Could you check a few things on this model? Use its own coordinates, in mm. Face numbers are marked on the shaded views. A direction names the side the tool comes from. Coordinates: 2 decimals unless noted, no trailing zeros. Order: outer loops, then holes, each group sorted by start corner. A loop starts at its lowest first (then second) coordinate and runs counter-clockwise, first axis right, second up. Notation, with made-up numbers: (-21, 45) - (17, 45) arc R24 cw to (17, 78) - close; hole circle Ø10 at (85, 10.25). An arc over 180 degrees is marked (long way). One line per item, written item: value.
Autodesk Inventor part; units mm, degrees
ref_plane "YZ Plane" through (0, 0, 0) normal (1, 0, 0) x (0, 1, 0)
ref_plane "XZ Plane" through (0, 0, 0) normal (0, 1, 0) x (-1, 0, 0)
ref_plane "XY Plane" through (0, 0, 0) normal (0, 0, 1) x (1, 0, 0)
sketch "Эскиз1" plane through (0, 0, 0) normal (0, 0, 1) x (1, 0, 0)
  circle A0 centre (0, 0) radius 2.1
  line L0 (-5, 14.35) -> (5, 14.35)
  line L1 (5, 14.35) -> (5, -14.35)
  line L2 (5, -14.35) -> (-5, -14.35)
  line L3 (-5, -14.35) -> (-5, 14.35)
  line L4 (-5, 14.35) -> (5, -14.35) construction
  line L5 (5, 14.35) -> (-5, -14.35) construction
  line L6 (-5, 7) -> (5, 7)
  dimension "d0" = 4.2
  dimension "d2" = 10
  dimension "d3" = 28.7
  dimension "d4" = 7
extrude "Выдавливание1" add sketch "Эскиз1" along normal blind 3.2 contours L6 L1 L2 L3
sketch "Эскиз2" plane through (0, 0, 3.2) normal (0, 0, 1) x (1, 0, 0)
  line L0 (5, -14.35) -> (5, 7)
  line L1 (5, -14.35) -> (-5, -14.35)
  line L2 (-5, -14.35) -> (-5, -11.15)
  line L3 (-5, -11.15) -> (5, -11.15)
  line L4 (5, -11.15) -> (5, -14.35)
  point P0 (0, 0)
  point P1 (5, -11.15)
  dimension "d7" = 10
  dimension "d8" = 3.2
extrude "Выдавливание2" add sketch "Эскиз2" along normal blind 13
fillet "Сопряжение1" radius 3 1 edges at (0, -11.15, 3.2)
sketch "Эскиз3" plane through (-5, -11.15, 16.2) normal (0, 1, 0) x (1, 0, 0)
  line L0 (0, 10) -> (10, 10)
  line L1 (5, 10) -> (5, 0)
  line L2 (0, 0) -> (10, 0)
  circle A0 centre (5, 5) radius 2.1
  point P0 (5, 16.2)
  dimension "d12" = 4.2
extrude "Выдавливание3" cut sketch "Эскиз3" against normal blind 13
sketch "Эскиз4" plane through (5, -14.35, 0) normal (1, 0, 0) x (0, 0, -1)
  line L0 (0, 0) -> (0, 21.35)
  line L1 (0, 21.35) -> (-3.2, 21.35)
  line L2 (-3.2, 6.2) -> (-3.2, 21.35)
  arc A0 (-6.2, 3.2) -> (-3.2, 6.2) centre (-6.2, 6.2) ccw
  line L3 (-6.2, 3.2) -> (-16.2, 3.2)
  line L4 (-16.2, 0) -> (-16.2, 3.2)
  line L5 (0, 0) -> (-16.2, 0)
  point P0 (0, 14.35)
extrude "Выдавливание4" add sketch "Эскиз4" along normal blind 3
sketch "Эскиз5" plane through (-5, -14.35, 0) normal (-1, 0, 0) x (0, 0, 1)
  line L0 (0, 21.35) -> (0, 0)
  line L1 (0, 0) -> (16.2, 0)
  line L2 (16.2, 3.2) -> (16.2, 0)
  line L3 (6.2, 3.2) -> (16.2, 3.2)
  arc A0 (3.2, 6.2) -> (6.2, 3.2) centre (6.2, 6.2) ccw
  line L4 (3.2, 21.35) -> (3.2, 6.2)
  line L5 (0, 21.35) -> (3.2, 21.35)
  point P0 (0, 14.35)
extrude "Выдавливание5" add sketch "Эскиз5" along normal blind 3
sketch "Эскиз6" plane through (8, -14.35, 0) normal (1, 0, 0) x (0, 0, -1)
  line L0 (-16.2, 3.2) -> (-16.2, 0)
  line L1 (-3.2, 21.35) -> (-16.2, 3.2)
  line L2 (-1.574, 20.1854) -> (-14.2, 2.5576)
  line L3 (-14.2, 2.5576) -> (-14.2, 0)
  line L4 (0, 0) -> (-16.2, 0)
  line L5 (0, 0) -> (0, 21.35)
  line L6 (0, 21.35) -> (-3.2, 21.35)
  line L7 (-3.2, 21.35) -> (-3.2, 6.2)
  arc A0 (-6.2, 3.2) -> (-3.2, 6.2) centre (-6.2, 6.2) ccw
  line L8 (-6.2, 3.2) -> (-16.2, 3.2)
  line L9 (-16.2, 3.2) -> (-16.2, 0)
  line L10 (-16.2, 0) -> (0, 0)
  point P0 (0, 14.35)
  point P1 (-13.7399, 3.2)
  point P2 (-3.2, 17.9153)
  dimension "d19" = 2
extrude "Выдавливание6" add sketch "Эскиз6" against normal blind 2 contours L1 L7 L2 L8
sketch "Эскиз7" plane through (-8, -14.35, 0) normal (-1, 0, 0) x (0, 0, 1)
  line L0 (16.2, 3.2) -> (13.7399, 3.2)
  line L1 (16.2, 3.2) -> (3.2, 21.35)
  line L2 (3.2, 17.9153) -> (3.2, 21.35)
  line L3 (3.2, 17.9153) -> (13.7399, 3.2)
  point P0 (0, 14.35)
extrude "Выдавливание7" add sketch "Эскиз7" against normal blind 2
properties part number "мертвое колесо крепл 25-26"
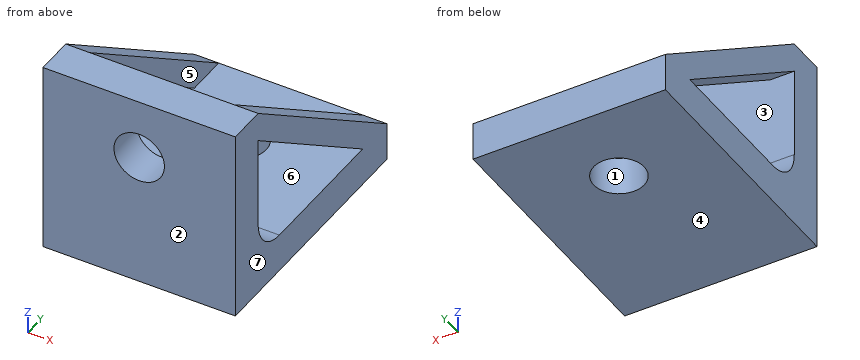
Item 1: If I drill on probe 1 along Y at (x, z) = (0, 0.8); probe 2 along X at (y, z) = (-13.7, 11.2); probe 3 along Y at (x, z) = (4.75, 8.25), over which ranges is the centre line in solid material (lowest first)?
Conclusion:
probe 1: -14.35 to -2.1, 2.1 to 7
probe 2: -8 to -2.1, 2.1 to 8
probe 3: -14.35 to -11.15
Item 2: I want a section at D-D on x = 6.5. Please give me the cut outline in (y, z).
Conclusion:
outline: (-14.35, 0) - (7, 0) - (7, 3.2) - (-11.15, 16.2) - (-14.35, 16.2) - close; hole (-11.15, 6.2) arc R3 ccw to (-8.15, 3.2) - (3.57, 3.2) - (-11.15, 13.74) - close
Item 3: I want a section at A-A on x = 0. Please give me the cut outline in (y, z).
Conclusion:
outline: (-14.35, 0) - (-2.1, 0) - (-2.1, 3.2) - (-8.15, 3.2) arc R3 cw to (-11.15, 6.2) - (-11.15, 9.1) - (-14.35, 9.1) - close; (-14.35, 13.3) - (-11.15, 13.3) - (-11.15, 16.2) - (-14.35, 16.2) - close; (2.1, 0) - (7, 0) - (7, 3.2) - (2.1, 3.2) - close
Item 4: For the marked faces 5, 6 and 7, which set-ups out of +Z, -Z, +X, -X, +Y, -Y let a thin tool reach every point of the face, with its end or its side?
Conclusion:
face 5: +Z, +Y
face 6: none
face 7: +Z, -Z, +X, +Y, -Y
Item 5: Thinking about a two-plate mould opening in Y: for the marked faces 1, 2, 3 and 4, which applies, pulls with the +Y half, pulls with the -Y half, needs draft (parallel to the pull), parting line crosses it, or undercut?
Conclusion:
face 1: undercut
face 2: pulls with the -Y half
face 3: undercut
face 4: needs draft
Item 6: I'm going to push flat-ended pins straight in: pin 1 Ø1.5 at (x, z) = (-0.5, 14) entering from +Y; pin 2 Ø2 at (x, y) = (-3.5, -0.5) entering from -Z; pin 3 Ø3.5 at (x, y) = (0, 0) entering from -Z. Where does each tip first touch, or does it pass through?
Conclusion:
pin 1: y = -11.15
pin 2: z = 0
pin 3: through
Item 7: I want a section at C-C on y = -9.5. Please give me the cut outline in (x, z).
Conclusion:
outline: (-8, 0) - (8, 0) - (8, 3.52) - (-8, 3.52) - close; (-8, 12.56) - (-6, 12.56) - (-6, 15.02) - (-8, 15.02) - close; (6, 12.56) - (8, 12.56) - (8, 15.02) - (6, 15.02) - close
Item 8: I want a section at B-B on z = 5.5. Please give me the cut outline in (x, y).
Conclusion:
outline: (-8, -14.35) - (8, -14.35) - (8, -11.07) - (-8, -11.07) - close; (-8, 0.35) - (-6, 0.35) - (-6, 3.79) - (-8, 3.79) - close; (6, 0.35) - (8, 0.35) - (8, 3.79) - (6, 3.79) - close
